Can you work these out from the model? Positions are in its coordinate system, mm. Give positions to 0.01 mm unless a question says otherwise; leave off trailing zeros. Order: outer loops, then holes, each group sorted by start corner. A loop starts at its lowest first (then second) coordinate and runs counter-clockwise, first axis right, second up. Notation, with made-up numbers: M -35,81.25 L -1,81.25 A23 cw -1,120.25 Z; hole C -4.75,-23 d5. An arc over 180 degrees is marked long. Write each question's results on one line, items separated by ' | '.
from build123d import *


with BuildPart() as part:
    # Esboço1 → Revolução1 (revolve)
    with BuildSketch(Plane(origin=(0, 0, 0), x_dir=(0, 0, -1), z_dir=(1, 0, 0))):
        with BuildLine():
            Line((0, 0), (-2, 0))
            ThreePointArc((-2, 0), (-3.060660172, 0.439339828), (-3.5, 1.5))
            Line((-3.5, 1.5), (-2, 1.5))
            Line((-2, 1.5), (-2, 4))
            Line((-2, 4), (-2.25, 4))
            Line((-2.25, 4), (-2.25, 9))
            Line((-2.25, 9), (0, 9))
            Line((0, 9), (0, 0))
        make_face()
    revolve(axis=Axis((0, 0, 0), (0, -1, 0)))


solid = part.part
(1) Will these pins go through, and if not, where does the flat tip stop? P1, Ø1, axis at x = -1.5, y = 8, coming from the -Z side; P2, Ø1, axis at y = 4.5, z = 2.5, coming from the -X side; P3, Ø2, axis at y = 3.5, z = 1.5, coming from the +X side.
Data:
P1: stops at z = -2.02 | P2: stops at x = -1.03 | P3: stops at x = 2.16
(2) Imagine slicing it at C-C, the plane y = 6. Write out the boundary of the cut face in (x, z), plus the area to 3 significant figures.
Data:
outline: C 0,0 d4.5 | area: 15.9 mm2
(3) I need wall thicknesses on L1, parallel to X at y = 8.25, z = -0.75; L2, parallel to Z at x = -1, y = 2; L3, parallel to X at y = 0.75, z = 1. Which ranges of each line are inside material? Lowest first, please. Write a range as from..to.
Data:
L1: x = -2.12..2.12 | L2: z = -1.73..1.73 | L3: x = -3.14..3.14
(4) Imagine slicing it at A-A, the plane x = 0. Write out the boundary of the cut face in (y, z), plus the area to 3 significant figures.
Data:
outline: M 0,-2 A1.5 ccw 1.5,-3.5 L 1.5,-2 L 4,-2 L 4,-2.25 L 9,-2.25 L 9,2.25 L 4,2.25 L 4,2 L 1.5,2 L 1.5,3.5 A1.5 ccw 0,2 Z | area: 42.0 mm2
(5) We'd pull the mould along Y, two halves only. Please class faces 1 (the face through (0, 9, 0)), 2 (the face through (2, 3, 0)), 3 (the face through (0, 0, 0)), 4 (the face through (-2.23, 6.54, -0.29)): +Y half, -Y half, draft (parallel to the pull), parting line (faces both ways), or undercut.
Data:
face 1: +Y half | face 2: undercut | face 3: -Y half | face 4: draft
(6) Imagine slicing it at D-D, the plane y = 3.5. Write out the boundary of the cut face in (x, z).
Data:
outline: C 0,0 d4
(7) Imagine slicing it at B-B, the plane z = 0. Write out the boundary of the cut face in (x, y), plus the area to 3 significant figures.
Data:
outline: M -3.5,1.5 A1.5 ccw -2,0 L 2,0 A1.5 ccw 3.5,1.5 L 2,1.5 L 2,4 L 2.25,4 L 2.25,9 L -2.25,9 L -2.25,4 L -2,4 L -2,1.5 Z | area: 42.0 mm2
